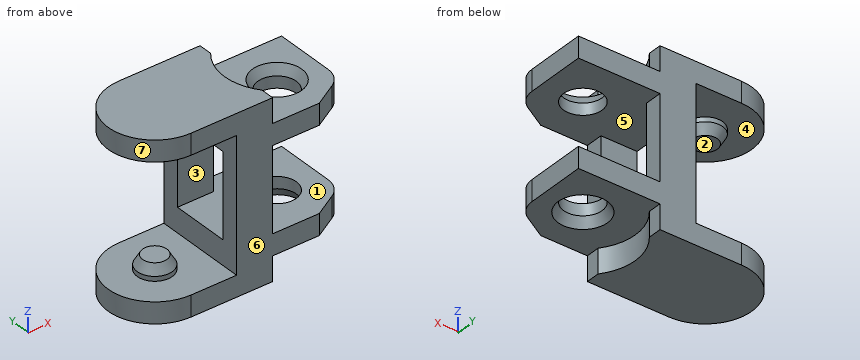
```python
from build123d import *

# Parameters (mm, degrees)
RESSALTO_EXTRUS_O1_DEPTH   = 7.5
ESBO_O2_W                  = 7.9
ESBO_O2_H                  = 11.4
ESBO_O2_W_2                = 7
ESBO_O2_H_2                = 2.1
ESBO_O2_H_3                = 7.2
CORTE_EXTRUS_O1_DEPTH      = 1
CORTE_EXTRUS_O1_DEPTH_BACK = 9
ESBO_O3_W                  = 7.2
ESBO_O3_H                  = 5
CORTE_EXTRUS_O2_DEPTH      = 8
CORTE_EXTRUS_O2_DEPTH_BACK = 12
ESBO_O4_R                  = 1.65
CORTE_EXTRUS_O3_DEPTH      = 3.1
CORTE_EXTRUS_O3_DEPTH_BACK = 13.9
ESBO_O5_R                  = 1.5
RESSALTO_EXTRUS_O2_DEPTH   = 1.2
ESBO_O6_R                  = 4.5
CORTE_EXTRUS_O4_DEPTH      = 2.1
FILETE1_R                  = 2
CHANFRO1_SIZE              = 0.8
CHANFRO1_SIZE2             = 0.461880215
CHANFRO1_PART_2_SIZE       = 0.8
CHANFRO1_PART_2_SIZE2      = 0.461880215
CHANFRO1_PART_3_SIZE       = 0.8
CHANFRO1_PART_3_SIZE2      = 0.461880215
CHANFRO1_PART_4_SIZE       = 0.8
CHANFRO1_PART_4_SIZE2      = 0.461880215


with BuildPart() as part:
    # Esboço1 → Ressalto-extrusão1 (new body, symmetric)
    with BuildSketch(Plane.XY):
        with BuildLine():
            Line((-7, 0), (7, 0))
            Line((7, 0), (7, -6.267949192))
            Line((7, -6.267949192), (4, -8))
            Line((4, -8), (-7, -8))
            ThreePointArc((-7, -8), (-11, -4), (-7, 0))
        make_face()
    extrude(amount=RESSALTO_EXTRUS_O1_DEPTH, both=True)

    # Esboço2 → Corte-extrusão1 (cut, two sides)
    with BuildSketch(Plane(origin=(0, 0, 0), x_dir=(1, 0, 0), z_dir=(0, 1, 0))) as corte_extrus_o1_sk:
        with Locations((-7.05, 0)):
            Rectangle(ESBO_O2_W, ESBO_O2_H)
        with Locations((3.5, -6.45)):
            Rectangle(ESBO_O2_W_2, ESBO_O2_H_2)
        with Locations((3.5, 6.45)):
            Rectangle(ESBO_O2_W_2, ESBO_O2_H_2)
        with Locations((3.5, 0)):
            Rectangle(ESBO_O2_W_2, ESBO_O2_H_3)
    extrude(amount=CORTE_EXTRUS_O1_DEPTH, mode=Mode.SUBTRACT)
    extrude(corte_extrus_o1_sk.sketch, amount=-CORTE_EXTRUS_O1_DEPTH_BACK, mode=Mode.SUBTRACT)

    # Esboço3 → Corte-extrusão2 (cut, two sides)
    with BuildSketch(Plane(origin=(0, 0, 0), x_dir=(0, 0, -1), z_dir=(1, 0, 0))) as corte_extrus_o2_sk:
        with Locations((0, -4)):
            Rectangle(ESBO_O3_W, ESBO_O3_H)
    extrude(amount=CORTE_EXTRUS_O2_DEPTH, mode=Mode.SUBTRACT)
    extrude(corte_extrus_o2_sk.sketch, amount=-CORTE_EXTRUS_O2_DEPTH_BACK, mode=Mode.SUBTRACT)

    # Esboço4 → Corte-extrusão3 (cut, two sides)
    with BuildSketch(Plane(origin=(0, 0, -5.4), x_dir=(-1, 0, 0), z_dir=(0, 0, -1))) as corte_extrus_o3_sk:
        with Locations((-3.5, -4)):
            Circle(ESBO_O4_R)
    extrude(amount=CORTE_EXTRUS_O3_DEPTH, mode=Mode.SUBTRACT)
    extrude(corte_extrus_o3_sk.sketch, amount=-CORTE_EXTRUS_O3_DEPTH_BACK, mode=Mode.SUBTRACT)

    # Esboço5 → Ressalto-extrusão2 (add)
    with BuildSketch(Plane(origin=(0, 0, 5.7), x_dir=(-1, 0, 0), z_dir=(0, 0, -1))):
        with Locations((7, -4)):
            Circle(ESBO_O5_R)
    ressalto_extrus_o2 = extrude(amount=RESSALTO_EXTRUS_O2_DEPTH)

    # Esboço6 → Corte-extrusão4 (cut)
    with BuildSketch(Plane.XY.offset(7.5)):
        with Locations((3.5, -4)):
            Circle(ESBO_O6_R)
    corte_extrus_o4 = extrude(amount=-CORTE_EXTRUS_O4_DEPTH, mode=Mode.SUBTRACT)

    # Espelhar1: Ressalto-extrusão2, Corte-extrusão4 across plane
    add(ressalto_extrus_o2.mirror(Plane.XY))
    add(corte_extrus_o4.mirror(Plane.XY), mode=Mode.SUBTRACT)

    # Filete1
    filete1_edges = [part.edges().sort_by_distance(p)[0] for p in [
        (7, -6.267949192, 4.5),
        (7, -6.267949192, -4.5),
    ]]
    fillet(filete1_edges, radius=FILETE1_R)

    # Chanfro1
    chanfro1_edges = [part.edges().sort_by_distance(p)[0] for p in [
        (5.15, -4, -5.4),
    ]]
    chanfro1_side = [part.faces().sort_by_distance(p)[0] for p in [
        (5.15, -4, -4.5),
    ]]
    chamfer(chanfro1_edges, length=CHANFRO1_SIZE, length2=CHANFRO1_SIZE2, reference=chanfro1_side[0])

    # Chanfro1 part 2
    chanfro1_part_2_edges = [part.edges().sort_by_distance(p)[0] for p in [
        (5.15, -4, 5.4),
    ]]
    chanfro1_part_2_side = [part.faces().sort_by_distance(p)[0] for p in [
        (5.15, -4, 4.5),
    ]]
    chamfer(chanfro1_part_2_edges, length=CHANFRO1_PART_2_SIZE, length2=CHANFRO1_PART_2_SIZE2, reference=chanfro1_part_2_side[0])

    # Chanfro1 part 3
    chanfro1_part_3_edges = [part.edges().sort_by_distance(p)[0] for p in [
        (-5.5, -4, 4.5),
    ]]
    chanfro1_part_3_side = [part.faces().sort_by_distance(p)[0] for p in [
        (-5.5, -4, 5.1),
    ]]
    chamfer(chanfro1_part_3_edges, length=CHANFRO1_PART_3_SIZE, length2=CHANFRO1_PART_3_SIZE2, reference=chanfro1_part_3_side[0])

    # Chanfro1 part 4
    chanfro1_part_4_edges = [part.edges().sort_by_distance(p)[0] for p in [
        (-5.5, -4, -4.5),
    ]]
    chanfro1_part_4_side = [part.faces().sort_by_distance(p)[0] for p in [
        (-5.5, -4, -5.1),
    ]]
    chamfer(chanfro1_part_4_edges, length=CHANFRO1_PART_4_SIZE, length2=CHANFRO1_PART_4_SIZE2, reference=chanfro1_part_4_side[0])


solid = part.part
```
Could you check a few things on this model? Use its own coordinates, in mm. Face numbers are marked on the shaded views. A direction names the side the tool comes from. Round coordinates to 2 decimals unless told otherwise and drop trailing zeros. Loops run counter-clockwise (first coordinate to the right, second up) from the corner with the lowest first, then second, coordinate; pieces in that order, holes last. Notation, with made-up numbers: (-22.75, -20.5) - (-14.75, -20.5) arc R7 cw to (-14.75, -7.5) - close; hole circle Ø9 at (34, 3.5). An arc over 180 degrees is marked (long way). Answer in a Markdown table with one row per item. Add a question column.
(1) For the marked faces 1, 2 and 3, which set-ups out of +Z, -Z, +X, -X, +Y, -Y let a thin tool reach every point of the face, with its end or its side?
(2) If we mould it in two halves opening along Y, with no side actions, what happens to the marked faces 4, 5, 6 and 7? For each: pulls with the +Y half, pulls with the -Y half, needs draft (parallel to the pull), parting line crosses it, or undercut.
(3) I'm going to push flat-ended pins straight in: pin 1 (0.6 mm diameter, centred on y = -1, z = -6.5, fed in from +X); pin 2 (2.5 mm diameter, centred on x = 4, y = -5, fed in from -Z); pin 3 (4 mm diameter, centred on x = 3, y = -3.5, fed in from +Z). Where does each tip first touch, or does it pass through?
(4) If we section it at D-D (y = -4): State how many separate pieces and enclosed holes the cut face has, plus the area to 3 significant figures.
(5) I need wall thicknesses on line 1 along Y through (x, z) = (3.5, -4.05); line 2 along Z through (x, y) = (-7, -5); line 3 along Z through (x, y) = (0, -4). Which ranges of each line are inside material? Lowest first, please.
(6) If we section it at B-B (x = 3.5): Please give me the cut outline in (y, z).
(7) If we section it at C-C (x = -3.5): Please give me the cut outline in (y, z), plus the area to 3 significant figures.
(8) If we section it at A-A (z = 2): Please give me the cut outline in (x, y).
Model answer:
| question | item | result |
|---|---|---|
| 1 | face 1 | +X |
| 1 | face 2 | -X, +Y, -Y |
| 1 | face 3 | +X, -X |
| 2 | face 4 | needs draft |
| 2 | face 5 | undercut |
| 2 | face 6 | pulls with the -Y half |
| 2 | face 7 | parting line crosses it |
| 3 | pin 1 | stops at x = 0 |
| 3 | pin 2 | stops at z = -5.4 |
| 3 | pin 3 | stops at z = 5.4 |
| 4 | separate pieces | 4 |
| 4 | enclosed holes | 0 |
| 4 | area | 67.5 mm² |
| 5 | line 1 | y = -8 to -5.65, -2.35 to 0 |
| 5 | line 2 | z = -7.5 to -4.5, 4.5 to 7.5 |
| 5 | line 3 | z = -5.4 to -3.6, 3.6 to 5.4 |
| 6 | outline | (-8, -5.4) - (-6.11, -5.4) - (-5.65, -4.6) - (-5.65, -3.6) - (-8, -3.6) - close; (-8, 3.6) - (-5.65, 3.6) - (-5.65, 4.6) - (-6.11, 5.4) - (-8, 5.4) - close; (-2.35, -4.6) - (-1.89, -5.4) - (0, -5.4) - (0, -3.6) - (-2.35, -3.6) - close; (-2.35, 3.6) - (0, 3.6) - (0, 5.4) - (-1.89, 5.4) - (-2.35, 4.6) - close |
| 7 | outline | (-8, -7.5) - (0, -7.5) - (0, -5.7) - (-8, -5.7) - close; (-8, 5.7) - (0, 5.7) - (0, 7.5) - (-8, 7.5) - close |
| 7 | area | 28.8 mm² |
| 8 | outline | (-3.1, -8) - (0, -8) - (0, -6.5) - (-3.1, -6.5) - close; (-3.1, -1.5) - (0, -1.5) - (0, 0) - (-3.1, 0) - close |
